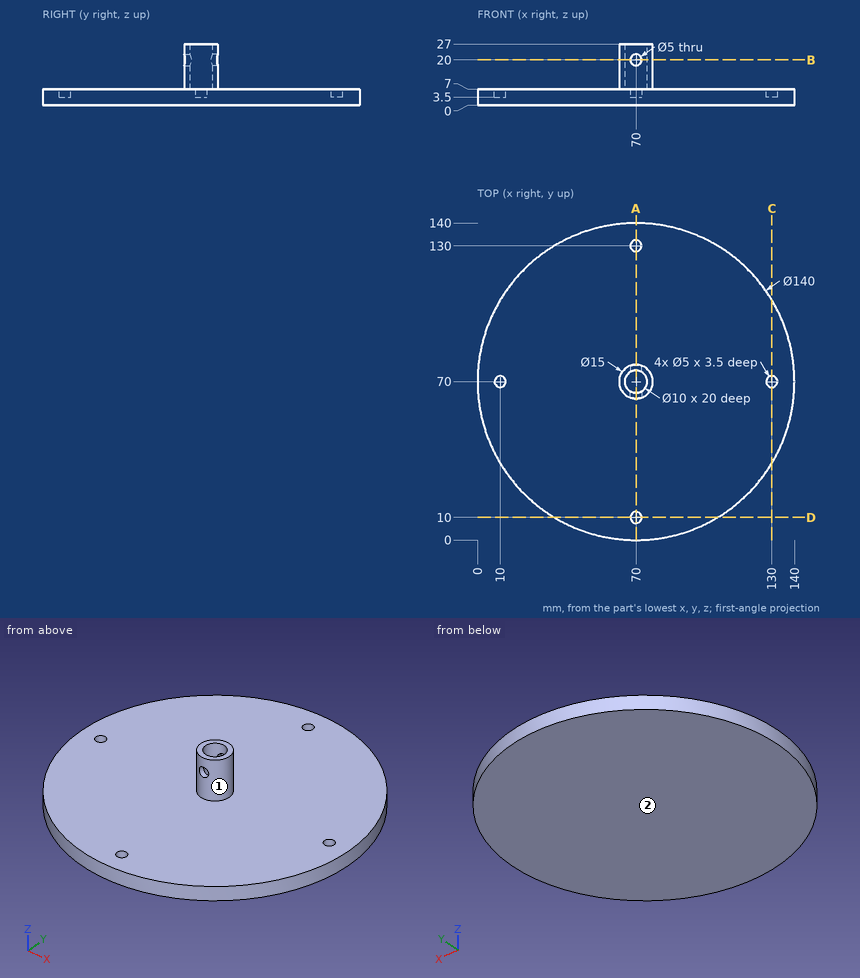
Design review of the part shown in the three views and the two pictorial views. Dimensions are in mm from the part's minimum x, y and z. A direction names the side the tool comes from. Round coordinates to 2 decimals unless told otherwise and drop trailing zeros. Loops run counter-clockwise (first coordinate to the right, second up) from the corner with the lowest first, then second, coordinate; pieces in that order, holes last. Notation, with made-up numbers: M 44,27 L 88,27 A19 ccw 88,54 Z; hole C 17,46 d9. An arc over 180 degrees is marked long. Write item = value, one per line.
Item 1: Take a section at C-C on x = 130. Write out the cut boundary in (y, z).
Return value:
outline = M 33.94,0 L 106.06,0 L 106.06,7 L 72.5,7 L 72.5,3.5 L 67.5,3.5 L 67.5,7 L 33.94,7 Z
Item 2: Machinability: for the marked faces 1 and 2, which of the approach directions +Z, -Z, +X, -X, +Y, -Y give a long, thin tool a straight path to every point of the face, cutting with its end or side? Answer none if there is none.
Return value:
face_1 = +Z
face_2 = -Z, +X, -X, +Y, -Y
Item 3: For line 1 (Y direction, x = 70, z = 4.6); line 2 (Z direction, x = 70, y = 64.3); line 3 (Y direction, x = 70, z = 15.5), list the stretches that pass through material, from the lowest coordinate up. Write a range as [from, to].
Return value:
line_1 = [0, 7.5], [12.5, 127.5], [132.5, 140]
line_2 = [0, 17.5], [22.5, 27]
line_3 = [62.5, 65], [75, 77.5]
Item 4: Take a section at A-A on x = 70. Write out the cut boundary in (y, z), then the cut area to 3 significant figures.
Return value:
outline = M 0,0 L 140,0 L 140,7 L 132.5,7 L 132.5,3.5 L 127.5,3.5 L 127.5,7 L 77.5,7 L 77.5,17.5 L 75,17.5 L 75,7 L 65,7 L 65,17.5 L 62.5,17.5 L 62.5,7 L 12.5,7 L 12.5,3.5 L 7.5,3.5 L 7.5,7 L 0,7 Z; M 62.5,22.5 L 65,22.5 L 65,27 L 62.5,27 Z; M 75,22.5 L 77.5,22.5 L 77.5,27 L 75,27 Z
area = 1,020 mm2
Item 5: Insertion check: P1, Ø5.5, axis at x = 71, y = 10, coming from the +Z side; P2, Ø4, axis at y = 77, z = 14.5, coming from the -X side; P3, Ø6.5, axis at x = 70, z = 20, coming from the -Y side. Each pin has a flat end and moves straight along its axis. Give the tip position at first contact, or say it passes through.
Return value:
P1 = 7
P2 = 64.41
P3 = 62.5
Item 6: Take a section at B-B on z = 20. Write out the cut boundary in (x, y), then the cut area to 3 significant figures.
Return value:
outline = M 67.5,62.93 L 67.5,65.67 A5 cw 67.5,74.33 L 67.5,77.07 A7.5 ccw Z; M 72.5,62.93 A7.5 ccw 72.5,77.07 L 72.5,74.33 A5 cw 72.5,65.67 Z
area = 72.4 mm2
